Autodesk Inventor part; units mm, degrees
ref_plane "YZ Plane" through (0, 0, 0) normal (1, 0, 0) x (0, 1, 0)
ref_plane "XZ Plane" through (0, 0, 0) normal (0, 1, 0) x (-1, 0, 0)
ref_plane "XY Plane" through (0, 0, 0) normal (0, 0, 1) x (1, 0, 0)
sketch "Sketch1" plane through (0, 0, 0) normal (0, 1, 0) x (-1, 0, 0)
  line L0 (0, 0) -> (25.4, 0)
  line L1 (25.4, 0) -> (25.4, -58.42)
  line L2 (25.4, -58.42) -> (0, -58.42)
  line L3 (0, -58.42) -> (0, 0)
  dimension "d0" = 25.4
  dimension "d1" = 58.42
extrude "Extrusion1" add sketch "Sketch1" along normal blind 3.81
sketch "Sketch2" plane through (0, 3.81, 0) normal (0, 1, 0) x (1, 0, 0)
  line L0 (-3.81, 3.81) -> (-21.59, 3.81)
  line L1 (-21.59, 3.81) -> (-21.59, 54.61)
  line L2 (-21.59, 54.61) -> (-3.81, 54.61)
  line L3 (-3.81, 54.61) -> (-3.81, 3.81)
  line L4 (-25.4, 58.42) -> (-25.4, 0)
  line L5 (-25.4, 0) -> (0, 0)
  line L6 (0, 0) -> (0, 58.42)
  line L7 (0, 58.42) -> (-25.4, 58.42)
  dimension "d4" = 17.78
  dimension "d5" = 50.8
extrude "Extrusion2" add sketch "Sketch2" along normal blind 25.4
sketch "Sketch3" plane through (0, 3.81, 0) normal (0, 1, 0) x (1, 0, 0)
  point P0 (0, 0)
  point P1 (-12.7, 16.51)
  point P2 (-12.7, 41.91)
hole "Hole1" at (-12.7, 3.81, -16.51) at (-12.7, 3.81, -41.91) direction (0, -1, 0) diameter 6.35 end through all countersink diameter 12.065 countersink angle 82
properties part number "batteryholder"
CAD build for the part. Positions are in the model's coordinates, mm. A direction names the side the tool comes from. Give positions to 0.01 mm unless a question says otherwise; leave off trailing zeros. Write each loop counter-clockwise with the first axis right and the second up, starting at its lowest first coordinate (ties: lowest second). Pieces come first, ordered by that corner, then holes. Notation, with made-up numbers: (-0.5, -3) -> (8.5, -3) arc R13 cw to (8.5, 8) -> close; hole circle Ø6 at (-6.75, 52.5). An arc over 180 degrees is marked (long way). Write each question's results on one line, items separated by ' | '.
1. Which spindle directions (+Z, -Z, +X, -X, +Y, -Y) get a long thin tool onto all of the face, cutting with end or side? Do faces 1 (the flat face through (-2, 29.21, -30)), 2 (the flat face through (-13, 16, -3.81)). Say none if no direction does.
Geometry check:
face 1: +Z, -Z, +X, -X, +Y | face 2: +Y
2. Wall check: probe 1 along Z at (x, y) = (-12.7, 0.1) (3 decimals); probe 2 along X at (y, z) = (0.25, -41.91) (3 decimals); probe 3 along Z at (x, y) = (-15.25, 20.5). Give the ranges that are in metal, low to high. Write a range as [from, to].
Geometry check:
probe 1: [-58.42, -45.085], [-38.735, -19.685], [-13.335, 0] | probe 2: [-25.4, -15.875], [-9.525, 0] | probe 3: [-58.42, -54.61], [-3.81, 0]
3. Cut at D-D, the plane x = -5.75. Write the cut outline in (y, z).
Geometry check:
outline: (0, -58.42) -> (29.21, -58.42) -> (29.21, -54.61) -> (3.81, -54.61) -> (3.81, -3.81) -> (29.21, -3.81) -> (29.21, 0) -> (0, 0) -> close
4. Cut at A-A, the plane z = -16.51. Write the cut outline in (x, y) (1 decimal), then the cut area to 3 significant figures.
Geometry check:
outline: (-25.4, 0) -> (-15.9, 0) -> (-15.9, 0.5) -> (-18.7, 3.8) -> (-21.6, 3.8) -> (-21.6, 29.2) -> (-25.4, 29.2) -> close; (-9.5, 0) -> (0, 0) -> (0, 29.2) -> (-3.8, 29.2) -> (-3.8, 3.8) -> (-6.7, 3.8) -> (-9.5, 0.5) -> close | area: 257 mm²
5. Cut at B-B, the plane y = 18. Write the cut outline in (x, z), then the cut area to 3 significant figures.
Geometry check:
outline: (-25.4, -58.42) -> (0, -58.42) -> (0, 0) -> (-25.4, 0) -> close; hole (-21.59, -54.61) -> (-3.81, -54.61) -> (-3.81, -3.81) -> (-21.59, -3.81) -> close | area: 581 mm²
6. Two-plate mould, pull along Z, no slides. Class faces 3 (the flat face through (-13, 14, 0)), 4 (the conical face through (-13.98, 0.73, -38.81)), 5 (the flat face through (0, 14, -30)): pulls with the +Z half, pulls with the -Z half, needs draft (parallel to the pull), parting line crosses it, or undercut.
Geometry check:
face 3: pulls with the +Z half | face 4: undercut | face 5: needs draft
7. Drop flat-ended pins along their axis: P1, Ø4, axis at x = -19.5, y = 21.5, coming from the +Z side; P2, Ø8.5, axis at x = -12.7, z = -16.51, coming from the +Y side; P3, Ø5.5, axis at x = -9, z = -20.5, coming from the +Y side; P4, Ø10, axis at x = -12.7, z = -41.91, coming from the +Y side. Give the stop position or say it passes through.
Geometry check:
P1: z = 0 | P2: y = 1.76 | P3: y = 3.81 | P4: y = 2.62
8. Cut at C-C, the plane x = -12.7. Write the cut outline in (y, z) (1 decimal).
Geometry check:
outline: (0, -58.4) -> (29.2, -58.4) -> (29.2, -54.6) -> (3.8, -54.6) -> (3.8, -47.9) -> (0.5, -45.1) -> (0, -45.1) -> close; (0, -38.7) -> (0.5, -38.7) -> (3.8, -35.9) -> (3.8, -22.5) -> (0.5, -19.7) -> (0, -19.7) -> close; (0, -13.3) -> (0.5, -13.3) -> (3.8, -10.5) -> (3.8, -3.8) -> (29.2, -3.8) -> (29.2, 0) -> (0, 0) -> close
